Build history of the part. All positions in model axes, mm. Face numbers are marked on the shaded views. Round coordinates to 2 decimals unless told otherwise and drop trailing zeros. Write each loop counter-clockwise with the first axis right and the second up, starting at its lowest first coordinate (ties: lowest second). Pieces come first, ordered by that corner, then holes. Notation, with made-up numbers: (35.5, 79.25) -> (48.5, 79.25) arc R30 cw to (48.5, 104.25) -> close; hole circle Ø2 at (25.5, -17.5). An arc over 180 degrees is marked (long way). Answer in a Markdown table with one row per item. Add a question column.
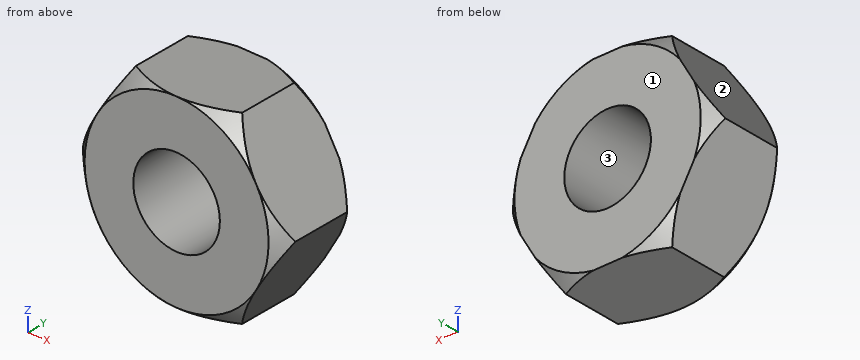
Autodesk Inventor part; units mm, degrees
ref_plane "YZ Plane" through (0, 0, 0) normal (1, 0, 0) x (0, 1, 0)
ref_plane "XZ Plane" through (0, 0, 0) normal (0, 1, 0) x (-1, 0, 0)
ref_plane "XY Plane" through (0, 0, 0) normal (0, 0, 1) x (1, 0, 0)
sketch "Sketch3" plane through (0, 0, 0) normal (0, 1, 0) x (-1, 0, 0)
  line L0 (-4.9048, -8.5016) -> (-9.815, -0.0031)
  line L1 (-9.815, -0.0031) -> (-4.9102, 8.4984)
  line L2 (-4.9102, 8.4984) -> (4.9048, 8.5016)
  line L3 (4.9048, 8.5016) -> (9.815, 0.0031)
  line L4 (9.815, 0.0031) -> (4.9102, -8.4984)
  line L5 (4.9102, -8.4984) -> (-4.9048, -8.5016)
  point P0 (0, 0)
  point P1 (0, 0)
  dimension "d1" = 17
extrude "Extrusion1" add sketch "Sketch3" along normal blind 8
sketch "Sketch4" plane through (0, 8, 0) normal (0, 1, 0) x (1, 0, 0)
  circle A0 centre (0, 0) radius 8.6061
extrude "Extrusion2" cut sketch "Sketch4" against normal through all draft 45 keep common part
sketch "Sketch22" plane through (0, 0, 0) normal (0, -1, 0) x (1, 0, 0)
  circle A0 centre (0, 0) radius 8.5
  line L0 (6.6894, 5.4144) -> (8.0357, 3.0809)
extrude "Extrusion12" cut sketch "Sketch22" against normal blind 8 draft 45 keep common part
sketch "Sketch23" plane through (0, 0, 0) normal (0, -1, 0) x (1, 0, 0)
  circle A0 centre (0, 0) radius 4
  dimension "d111" = 8
extrude "Extrusion13" cut sketch "Sketch23" against normal blind 8
properties part number "Bolt"
(1) Drop flat-ended pins along their axis: P1, Ø2, axis at x = -2.5, y = 5.5, coming from the -Z side; P2, Ø1.5, axis at x = 6, y = 2, coming from the -Z side; P3, Ø3, axis at y = 5.5, z = -6, coming from the -X side; P4, Ø5, axis at x = 7.5, z = 5, coming from the +Y side. Give the stop position or say it passes through.
(2) Probe line 1 along Z through (x, y) = (0, 2.5); line 2 along X through (y, z) = (1.5, 1.5); line 3 along X through (y, z) = (4, 2). List the from-to ranges inside material, lowest first.
(3) Saw through at A-A (y = 2.5). List the corners of the cut face in (x, z) (3 decimals), plus the area to 3 significant figures.
(4) Saw through at B-B (y = 0.5). List the corners of the cut face in (x, z).
(5) Mould opens along Z. For the marked faces 1, 2 and 3 say: pulls with the +Z half, pulls with the -Z half, needs draft (parallel to the pull), parting line crosses it, or undercut.
Answer sheet:
| question | item | result |
|---|---|---|
| 1 | P1 | stops at z = -8.5 |
| 1 | P2 | stops at z = -7.9 |
| 1 | P3 | stops at x = -7.22 |
| 1 | P4 | stops at y = 8 |
| 2 | line 1 | z = -8.5 to -4, 4 to 8.5 |
| 2 | line 2 | x = -8.95 to -3.71, 3.71 to 8.95 |
| 2 | line 3 | x = -8.66 to -3.46, 3.46 to 8.66 |
| 3 | outline | (-9.815, 0.003) -> (-4.91, -8.498) -> (4.905, -8.502) -> (9.815, -0.003) -> (4.91, 8.498) -> (-4.905, 8.502) -> close; hole circle Ø8 at (0, 0) |
| 3 | area | 200 mm² |
| 4 | outline | (-8.84, -1.69) -> (-5.88, -6.81) arc R9 ccw to (-2.96, -8.5) -> (2.96, -8.5) arc R9 ccw to (5.88, -6.81) -> (8.84, -1.69) arc R9 ccw to (8.84, 1.69) -> (5.88, 6.81) arc R9 ccw to (2.96, 8.5) -> (-2.96, 8.5) arc R9 ccw to (-5.88, 6.81) -> (-8.84, 1.69) arc R9 ccw to start; hole circle Ø8 at (0, 0) |
| 5 | face 1 | needs draft |
| 5 | face 2 | pulls with the +Z half |
| 5 | face 3 | undercut |
